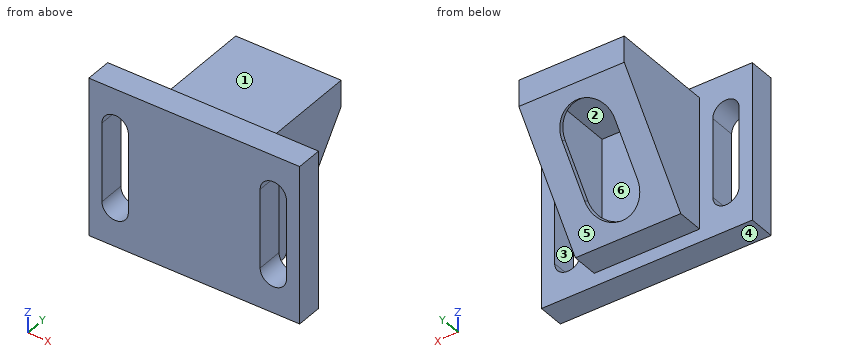
from build123d import *

# Parameters (mm, degrees)
SKETCH1_W           = 101.6
SKETCH1_H           = 76.2
BOSS_EXTRUDE1_DEPTH = 12.7
CUT_EXTRUDE1_DEPTH  = 12.7
BOSS_EXTRUDE2_DEPTH = 25.4
CUT_EXTRUDE3_DEPTH  = 12.7
CUT_EXTRUDE7_DEPTH  = 21.59


with BuildPart() as part:
    # Sketch1 → Boss-Extrude1 (new body)
    with BuildSketch(Plane(origin=(0, 0, 0), x_dir=(1, 0, 0), z_dir=(0, 1, 0))):
        with Locations((50.8, -38.1)):
            Rectangle(SKETCH1_W, SKETCH1_H)
    extrude(amount=BOSS_EXTRUDE1_DEPTH)

    # Sketch4 → Cut-Extrude1 (cut)
    with BuildSketch(Plane(origin=(0, 12.7, 0), x_dir=(1, 0, 0), z_dir=(0, 1, 0))):
        with BuildLine():
            Line((19.05, -19.05), (19.05, -57.15))
            ThreePointArc((19.05, -57.15), (12.7, -63.5), (6.35, -57.15))
            Line((6.35, -57.15), (6.35, -19.05))
            ThreePointArc((6.35, -19.05), (12.7, -12.7), (19.05, -19.05))
        make_face()
        with BuildLine():
            Line((95.25, -19.05), (95.25, -57.15))
            ThreePointArc((95.25, -57.15), (88.9, -63.5), (82.55, -57.15))
            Line((82.55, -57.15), (82.55, -19.05))
            ThreePointArc((82.55, -19.05), (88.9, -12.7), (95.25, -19.05))
        make_face()
    extrude(amount=-CUT_EXTRUDE1_DEPTH, mode=Mode.SUBTRACT)

    # Sketch5 → Boss-Extrude2 (add, symmetric)
    with BuildSketch(Plane(origin=(50.8, 0, 0), x_dir=(0, 0, -1), z_dir=(1, 0, 0))):
        Polygon((-6.35, 12.7), (-6.35, 25.4), (-57.15, 63.5), (-69.85, 63.5), (-69.85, 12.7), align=None)
    extrude(amount=BOSS_EXTRUDE2_DEPTH, both=True)

    # Sketch10 → Cut-Extrude3 (cut)
    with BuildSketch(Plane(origin=(0, 13.208, -9.906), x_dir=(1, 0, 0), z_dir=(0, 0.8, -0.5999999999999999))):
        with BuildLine():
            Line((63.5, -39.37), (63.5, -64.77))
            ThreePointArc((63.5, -64.77), (50.8, -77.47), (38.1, -64.77))
            Line((38.1, -64.77), (38.1, -39.37))
            ThreePointArc((38.1, -39.37), (50.8, -26.67), (63.5, -39.37))
        make_face()
    extrude(amount=-CUT_EXTRUDE3_DEPTH, mode=Mode.SUBTRACT)

    # Sketch12 → Cut-Extrude7 (cut, symmetric)
    with BuildSketch(Plane(origin=(50.8, 0, 0), x_dir=(0, 0, -1), z_dir=(1, 0, 0))):
        Polygon((-10.16, 25.0825), (-56.303333333, 59.69), (-69.596, 59.69), (-69.596, 12.7), (-10.16, 12.7), align=None)
    extrude(amount=CUT_EXTRUDE7_DEPTH, both=True, mode=Mode.SUBTRACT)


solid = part.part
For this review, take the finished solid that the model builds, in its own axes (mm). Face numbers are marked on the shaded views. A direction names the side the tool comes from. Coordinates: 2 decimals unless noted, no trailing zeros. Loops run counter-clockwise (first coordinate to the right, second up) from the corner with the lowest first, then second, coordinate; pieces in that order, holes last. Notation, with made-up numbers: (-23.5, 78.5) - (27.5, 78.5) arc R24 cw to (27.5, 108.5) - close; hole circle Ø4 at (15, 53). An arc over 180 degrees is marked (long way). Use a Markdown table: item, result. Add a question column.
Item 1: We need section C-C (z = 35.5). Give the boundary of the cut face in (x, y).
Item 2: Mouldability with a two-part tool opening along Y and no side actions: class the marked faces 4, 5 and 6 as pulls with the +Y half, pulls with the -Y half, needs draft (parallel to the pull), parting line crosses it, or undercut.
Item 3: For line 1 (X direction, y = 38.5, z = 59); line 2 (Z direction, x = 55, y = 15.5); line 3 (Y direction, x = 48, z = 12), list the stretches that pass through material, from the lowest coordinate up.
Item 4: We need section B-B (y = 19.5). Give the boundary of the cut face in (x, z).
Item 5: Insertion check: pin 1 Ø15 at (y, z) = (50, 49.5) entering from +X; pin 2 Ø3.5 at (x, y) = (48.5, 21) entering from +Z; pin 3 Ø10 at (x, z) = (18, 42.5) entering from +Y. Each pin has a flat end and moves straight along its axis. Give the tip position at first contact, or say it passes through.
Item 6: Tool access review of the marked faces 1, 2 and 3: name each direction out of +Z, -Z, +X, -X, +Y, -Y from which nothing blocks a thin tool from reaching the whole face with its end or side.
Item 7: We need section A-A (x = 88.9). Give the boundary of the cut face in (y, z).
Item 8: We need section D-D (x = 68.5). Give the boundary of the cut face in (y, z).
Results list:
| question | item | result |
|---|---|---|
| 1 | outline | (0, 0) - (6.35, 0) - (6.35, 12.7) - (0, 12.7) - close; (19.05, 0) - (82.55, 0) - (82.55, 12.7) - (76.2, 12.7) - (76.2, 47.26) - (63.5, 47.26) - (63.5, 44.09) - (72.39, 44.09) - (72.39, 12.7) - (29.21, 12.7) - (29.21, 44.09) - (38.1, 44.09) - (38.1, 47.26) - (25.4, 47.26) - (25.4, 12.7) - (19.05, 12.7) - close; (95.25, 0) - (101.6, 0) - (101.6, 12.7) - (95.25, 12.7) - close |
| 2 | face 4 | needs draft |
| 2 | face 5 | pulls with the +Y half |
| 2 | face 6 | undercut |
| 3 | line 1 | x = 25.4 to 29.21, 72.39 to 76.2 |
| 3 | line 2 | z = 6.35 to 10.16, 69.6 to 69.85 |
| 3 | line 3 | y = 0 to 12.7, 26.46 to 28.97 |
| 4 | outline | (25.4, 6.35) - (76.2, 6.35) - (76.2, 69.85) - (25.4, 69.85) - close; hole (29.21, 10.16) - (72.39, 10.16) - (72.39, 69.6) - (29.21, 69.6) - close |
| 5 | pin 1 | stops at x = 76.2 |
| 5 | pin 2 | stops at z = 69.85 |
| 5 | pin 3 | stops at y = 12.7 |
| 6 | face 1 | +Z, +X, -X, +Y |
| 6 | face 2 | none |
| 6 | face 3 | +Y, -Y |
| 7 | outline | (0, 0) - (12.7, 0) - (12.7, 12.7) - (0, 12.7) - close; (0, 63.5) - (12.7, 63.5) - (12.7, 76.2) - (0, 76.2) - close |
| 8 | outline | (0, 0) - (12.7, 0) - (12.7, 6.35) - (25.4, 6.35) - (63.5, 57.15) - (63.5, 69.85) - (12.7, 69.85) - (12.7, 76.2) - (0, 76.2) - close; hole (12.7, 10.16) - (25.08, 10.16) - (59.69, 56.3) - (59.69, 69.6) - (12.7, 69.6) - close |
